Source: CAD feature listing. Evaluate the final solid. Frame: model axes, mm. A direction names the side the tool comes from. Give positions to 0.01 mm unless a question says otherwise; leave off trailing zeros. Loops run counter-clockwise (first coordinate to the right, second up) from the corner with the lowest first, then second, coordinate; pieces in that order, holes last. Notation, with made-up numbers: (-10.75, -9) -> (35.25, -9) arc R29 ccw to (35.25, 25) -> close; hole circle Ø4 at (67, -22). An arc over 180 degrees is marked (long way). Put each result on its own line as item: value.
```python
from build123d import *

# Parameters (mm, degrees)
F0_R          = 10.5
F0_R_2        = 2.65
F1_DEPTH      = 18
F2_R          = 5
F3_DEPTH      = 7.8
F3_DEPTH_BACK = 7.8
F4_SIZE2      = 5
F4_SIZE       = 15


with BuildPart() as f1:
    # F0 (on Top) → F1 (new body)
    with BuildSketch(Plane.XY):
        Circle(F0_R)
        Circle(F0_R_2, mode=Mode.SUBTRACT)
    extrude(amount=F1_DEPTH)

    # F2 (on Right) → F3 (cut, two sides)
    with BuildSketch(Plane.YZ) as f3_sk:
        with Locations((0, 16.75)):
            Circle(F2_R)
    extrude(amount=-F3_DEPTH, mode=Mode.SUBTRACT)
    extrude(f3_sk.sketch, amount=F3_DEPTH_BACK, mode=Mode.SUBTRACT)

    # F4
    f4_edges = [f1.edges().sort_by_distance(p)[0] for p in [
        (-10.5, 0, 0),
    ]]
    f4_side = f1.faces().sort_by_distance((-10.5, 0, 9))[0]
    chamfer(f4_edges, length=F4_SIZE, length2=F4_SIZE2, reference=f4_side)


solid = f1.part
```
(1) Section D-D on z = 6. Return loops of the section in (x, y).
Calculated:
outline: circle Ø15 at (0, 0); hole circle Ø5.3 at (0, 0)
(2) Draft query along X for faces 3 (the flat face through (0, -7, 18)), 4 (the cylindrical face through (2.45, -1.01, 6.17)), 5 (the cylindrical face through (10, 3.2, 16.5)). Return one class per face: released by +X, released by -X, zero draft, split by the parting line, or undercut.
Calculated:
face 3: zero draft
face 4: undercut
face 5: split by the parting line
(3) Section C-C on x = 0. Return loops of the section in (y, z), then the cut area to 3 significant figures.
Calculated:
outline: (-10.5, 15) -> (-5.5, 0) -> (-2.65, 0) -> (-2.65, 12.51) arc R5 cw to (-4.84, 18) -> (-10.5, 18) -> close; (2.65, 0) -> (5.5, 0) -> (10.5, 15) -> (10.5, 18) -> (4.84, 18) arc R5 cw to (2.65, 12.51) -> close
area: 188 mm²
(4) Line query: probe 1 along X at (y, z) = (-1.75, 3.5); probe 2 along X at (y, z) = (-0.75, 4); probe 3 along Z at (x, y) = (4.5, 0). Output: solid intervals per line, ascending. Write a range as from..to.
Calculated:
probe 1: x = -6.43..-1.99, 1.99..6.43
probe 2: x = -6.79..-2.54, 2.54..6.79
probe 3: z = 0..11.75
(5) Section A-A on y = 0. Return loops of the section in (x, z).
Calculated:
outline: (-10.5, 15) -> (-5.5, 0) -> (-2.65, 0) -> (-2.65, 11.75) -> (-7.8, 11.75) -> (-7.8, 18) -> (-10.5, 18) -> close; (2.65, 0) -> (5.5, 0) -> (10.5, 15) -> (10.5, 18) -> (7.8, 18) -> (7.8, 11.75) -> (2.65, 11.75) -> close
(6) Reachability of faces 1 (the cylindrical face through (0.11, -3.71, 13.4)), 2 (the conical face through (-5.88, -4.51, 5.73)) from +Z, -Z, +X, -X, +Y, -Y: full face, straight path, thin tool, end or side. Return the list, or none.
Calculated:
face 1: none
face 2: -Z
(7) First-contact query: P1, Ø4, axis at x = 6, z = 5.5, coming from the +Y side; P2, Ø2, axis at x = 4, y = 3, coming from the +Z side; P3, Ø5, axis at x = -4, z = 6.5, coming from the -Y side. Flat tips, straight axial feed; report the tip coordinate or a pass-through.
Calculated:
P1: stops at y = 6.37
P2: stops at z = 13.75
P3: stops at y = -7.95
(8) Section B-B on z = 16.75. Return loops of the section in (x, y), then the cut area to 3 significant figures.
Calculated:
outline: circle Ø21 at (0, 0); hole (-7.8, -5) -> (7.8, -5) -> (7.8, 5) -> (-7.8, 5) -> close
area: 190 mm²
